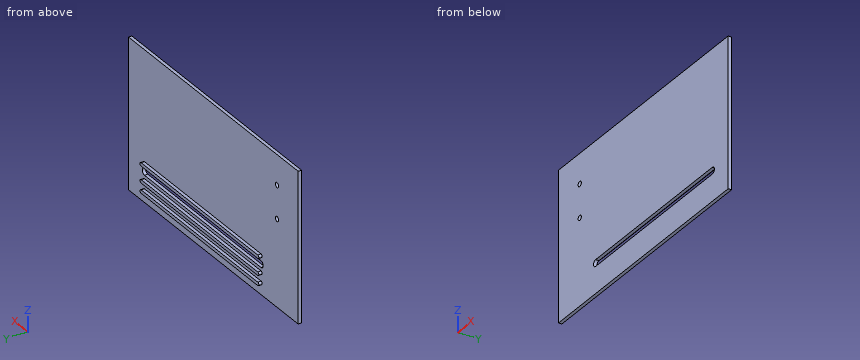
```python
from build123d import *

# Parameters (mm, degrees)
SKETCH1_W           = 800
SKETCH1_H           = 450
SKETCH1_R           = 7.5
BOSS_EXTRUDE1_DEPTH = 10
BOSS_EXTRUDE2_DEPTH = 10


with BuildPart() as part:
    # Sketch1 → Boss-Extrude1 (new body)
    with BuildSketch(Plane(origin=(0, 0, 0), x_dir=(1, 0, 0), z_dir=(0, 1, 0))):
        with Locations((400, 225)):
            Rectangle(SKETCH1_W, SKETCH1_H)
        with Locations(Location((100, 190, 0), (0, 0, 270))):
            Circle(SKETCH1_R, mode=Mode.SUBTRACT)
        with Locations(Location((100, 90, 0), (0, 0, 270))):
            Circle(SKETCH1_R, mode=Mode.SUBTRACT)
        with BuildLine():
            Line((175, 370), (725, 370))
            ThreePointArc((725, 370), (735, 360), (725, 350))
            Line((725, 350), (175, 350))
            ThreePointArc((175, 350), (165, 360), (175, 370))
        make_face(mode=Mode.SUBTRACT)
    extrude(amount=BOSS_EXTRUDE1_DEPTH)

    # Sketch2 → Boss-Extrude2 (add)
    with BuildSketch(Plane(origin=(0, 10, 0), x_dir=(1, 0, 0), z_dir=(0, 1, 0))):
        with BuildLine():
            Line((175, 390), (725, 390))
            ThreePointArc((725, 390), (730, 385), (725, 380))
            Line((725, 380), (175, 380))
            ThreePointArc((175, 380), (170, 385), (175, 390))
        make_face()
        with BuildLine():
            Line((175, 340), (725, 340))
            ThreePointArc((725, 340), (730, 335), (725, 330))
            Line((725, 330), (175, 330))
            ThreePointArc((175, 330), (170, 335), (175, 340))
        make_face()
        with BuildLine():
            Line((175, 420), (725, 420))
            ThreePointArc((725, 420), (730, 415), (725, 410))
            Line((725, 410), (175, 410))
            ThreePointArc((175, 410), (170, 415), (175, 420))
        make_face()
    extrude(amount=BOSS_EXTRUDE2_DEPTH)


solid = part.part
```
CAD build for the part. Positions are in the model's coordinates, mm. Give positions to 0.01 mm unless a question says otherwise; leave off trailing zeros. Order: outer loops, then holes, each group sorted by start corner. A loop starts at its lowest first (then second) coordinate and runs counter-clockwise, first axis right, second up.
(1) Drill centre lines: L1, parallel to Z at x = 499, y = 14.5; L2, parallel to X at y = 2, z = -90; L3, parallel to Z at x = 227.5, y = 1.25. Where is each one in solid material? Low to high.
(2) Flat gauge pins, fed straight in: pin 1 (3 mm diameter, centred on x = 506, y = 17, fed in from -Z); pin 2 (5 mm diameter, centred on x = 567, y = 13.5, fed in from +Z); pin 3 (2 mm diameter, centred on x = 631, z = -310.5, fed in from +Y). Where does each tip first touch, or does it go through?
(3) Saw through at D-D, the plane x = 100. Give the cut face in (y, z).
(4) Saw through at B-B, the plane z = -90. Give the cut face in (x, y).
(5) Saw through at C-C, the plane y = 7. Give the cut face in (x, z).
(6) Saw through at A-A, the plane x = 274.5. Give the cut face in (y, z).
Results found:
1. L1: z = -420 to -410, -390 to -380, -340 to -330
1. L2: x = 0 to 92.5, 107.5 to 800
1. L3: z = -450 to -370, -350 to 0
2. pin 1: stops at z = -420
2. pin 2: stops at z = -330
2. pin 3: stops at y = 10
3. outline: (0, -450) - (10, -450) - (10, -197.5) - (0, -197.5) - close; (0, -182.5) - (10, -182.5) - (10, -97.5) - (0, -97.5) - close; (0, -82.5) - (10, -82.5) - (10, 0) - (0, 0) - close
4. outline: (0, 0) - (92.5, 0) - (92.5, 10) - (0, 10) - close; (107.5, 0) - (800, 0) - (800, 10) - (107.5, 10) - close
5. outline: (0, -450) - (800, -450) - (800, 0) - (0, 0) - close; hole circle Ø15 at (100, -190); hole circle Ø15 at (100, -90); hole (175, -370) - (725, -370) arc R10 ccw to (725, -350) - (175, -350) arc R10 ccw to start
6. outline: (0, -450) - (10, -450) - (10, -420) - (20, -420) - (20, -410) - (10, -410) - (10, -390) - (20, -390) - (20, -380) - (10, -380) - (10, -370) - (0, -370) - close; (0, -350) - (10, -350) - (10, -340) - (20, -340) - (20, -330) - (10, -330) - (10, 0) - (0, 0) - close
